The figure shows three views and two pictorial views of one solid part (mm, origin at its lowest corner). Answer the questions. Coordinates: 2 decimals unless noted, no trailing zeros. Write each loop counter-clockwise with the first axis right and the second up, starting at its lowest first coordinate (ties: lowest second). Pieces come first, ordered by that corner, then holes. Notation, with made-up numbers: M 38.25,89.25 L 89.25,89.25 A19 ccw 89.25,124.25 Z; hole C -31.5,-8 d1. An arc over 180 degrees is marked long. Use CSV: the item, a comma, the result in double quotes.
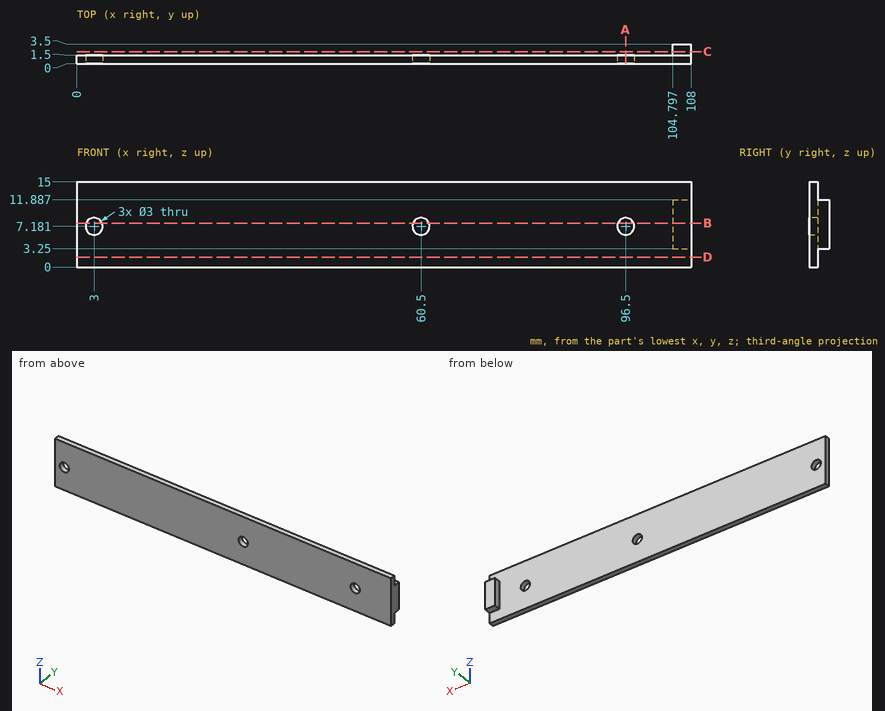
Item 1: The part is cut by section D-D (z = 1.75). Write down the section's boundary in (x, y).
Answer:
outline,"M 0,0 L 108,0 L 108,1.5 L 0,1.5 Z"
Item 2: The part is cut by section C-C (y = 2.15). Write down the section's boundary in (x, z).
Answer:
outline,"M 104.8,3.25 L 108,3.25 L 108,11.89 L 104.8,11.89 Z"
Item 3: Given pin 1 (7.5 mm diameter, centred on x = 78, z = 10, fed in from +Y); pin 2 (1 mm diameter, centred on y = 2.5, z = 9, fed in from -X); pin 3 (2 mm diameter, centred on x = 41, z = 4, fed in from -Y); pin 4 (1.6 mm diameter, centred on x = 106.5, y = 2.5, fed in from -Z), each flat-ended and moving along its own axis, determine where each tip first touches the part or whether it passes through.
Answer:
pin 1,"stops at y = 1.5"
pin 2,"stops at x = 104.8"
pin 3,"stops at y = 0"
pin 4,"stops at z = 3.25"
Item 4: Consider probe 1 along Z at (x, y) = (96.5, 0.8); probe 2 along Y at (x, z) = (28.5, 8.25); probe 3 along X at (y, z) = (1.45, 6.5). Determine where each line is inside the solid, lowest interval first.
Answer:
probe 1,"z = 0 to 5.68, 8.68 to 15"
probe 2,"y = 0 to 1.5"
probe 3,"x = 0 to 1.66, 4.34 to 59.16, 61.84 to 95.16, 97.84 to 108"
Item 5: The part is cut by section B-B (z = 7.75). Write down the section's boundary in (x, y).
Answer:
outline,"M 0,0 L 1.61,0 L 1.61,1.5 L 0,1.5 Z; M 4.39,0 L 59.11,0 L 59.11,1.5 L 4.39,1.5 Z; M 61.89,0 L 95.11,0 L 95.11,1.5 L 61.89,1.5 Z; M 97.89,0 L 108,0 L 108,3.5 L 104.8,3.5 L 104.8,1.5 L 97.89,1.5 Z"
Item 6: The part is cut by section A-A (x = 96.5). Write down the section's boundary in (y, z), then the cut area to 3 significant figures.
Answer:
outline,"M 0,0 L 1.5,0 L 1.5,5.68 L 0,5.68 Z; M 0,8.68 L 1.5,8.68 L 1.5,15 L 0,15 Z"
area,"18.0 mm2"
